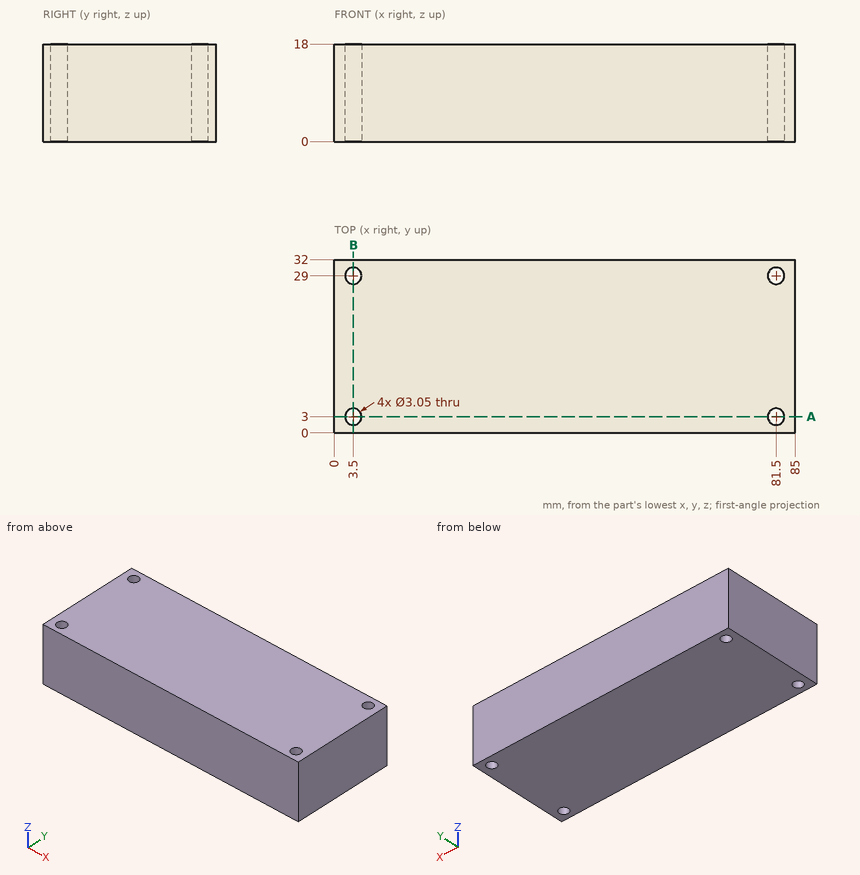
The figure shows three views and two pictorial views of one solid part (mm, origin at its lowest corner). Answer the questions. Round coordinates to 2 decimals unless told otherwise and drop trailing zeros. Order: outer loops, then holes, each group sorted by start corner. A loop starts at its lowest first (then second) coordinate and runs counter-clockwise, first axis right, second up.
Q1. A cutting plane is placed at B-B, the plane x = 3.5. Determine the outline of the cut face in (y, z) (3 decimals), then the cut area to 3 significant figures.
Solution:
outline: (0, 0) - (1.475, 0) - (1.475, 18) - (0, 18) - close; (4.525, 0) - (27.475, 0) - (27.475, 18) - (4.525, 18) - close; (30.525, 0) - (32, 0) - (32, 18) - (30.525, 18) - close
area: 466 mm2
Q2. A cutting plane is placed at A-A, the plane y = 3. Determine the outline of the cut face in (x, z) (3 decimals), then the cut area to 3 significant figures.
Solution:
outline: (0, 0) - (1.975, 0) - (1.975, 18) - (0, 18) - close; (5.025, 0) - (79.975, 0) - (79.975, 18) - (5.025, 18) - close; (83.025, 0) - (85, 0) - (85, 18) - (83.025, 18) - close
area: 1,420 mm2
Q3. Given pin 1 Ø2.5 at (x, y) = (81.5, 3) entering from -Z, flat-ended and moving along its own axis, determine where the tip first touches the part or whether it passes through.
Solution:
pin 1: passes through
Q4. Find the intervals of material crossed by line 1 along Y through (x, z) = (81.5, 7.5) (3 decimals), in increasing order.
Solution:
line 1: y = 0 to 1.475, 4.525 to 27.475, 30.525 to 32
